from build123d import *

# Parameters (mm, degrees)
SKIZZE1_W                       = 50
SKIZZE1_H                       = 29
SKIZZE1_R                       = 3
AUFSATZ_LINEAR_AUSTRAGEN1_DEPTH = 2
SKIZZE2_W                       = 30
SKIZZE2_H                       = 2
AUFSATZ_LINEAR_AUSTRAGEN2_DEPTH = 49.5
SKIZZE3_R                       = 1.5
SKIZZE3_R_2                     = 1.822550398
SKIZZE3_W                       = 4
SKIZZE3_H                       = 11
SKIZZE3_W_2                     = 6.639290737
SKIZZE3_H_2                     = 4.5
SCHNITT_LINEAR_AUSTRAGEN1_DEPTH = 49.5
SKIZZE4_W                       = 20
SKIZZE4_H                       = 12.5
SCHNITT_LINEAR_AUSTRAGEN2_DEPTH = 49.5


with BuildPart() as part:
    # Skizze1 → Aufsatz-Linear austragen1 (new body)
    with BuildSketch(Plane(origin=(0, 0, 0), x_dir=(1, 0, 0), z_dir=(0, 1, 0))):
        Rectangle(SKIZZE1_W, SKIZZE1_H)
        with Locations(Location((14.802393345, -9.5, 0), (0, 0, 270))):
            Circle(SKIZZE1_R, mode=Mode.SUBTRACT)
        with Locations(Location((-17.197606655, -9.5, 0), (0, 0, 270))):
            Circle(SKIZZE1_R, mode=Mode.SUBTRACT)
    extrude(amount=AUFSATZ_LINEAR_AUSTRAGEN1_DEPTH)

    # Skizze2 → Aufsatz-Linear austragen2 (add)
    with BuildSketch(Plane(origin=(0, 2, 0), x_dir=(1, 0, 0), z_dir=(0, 1, 0))):
        with Locations((-10, 13.5)):
            Rectangle(SKIZZE2_W, SKIZZE2_H)
    extrude(amount=AUFSATZ_LINEAR_AUSTRAGEN2_DEPTH)

    # Skizze3 → Schnitt-Linear austragen1 (cut)
    with BuildSketch(Plane.XY.offset(-12.5)):
        with Locations((-22, 49)):
            Circle(SKIZZE3_R)
        with Locations((-22, 34)):
            Circle(SKIZZE3_R)
        with Locations((0, 41.5)):
            Circle(SKIZZE3_R_2)
        with Locations((-23, 41.5)):
            Rectangle(SKIZZE3_W, SKIZZE3_H)
        with Locations((-11.748940962, 49.25)):
            Rectangle(SKIZZE3_W_2, SKIZZE3_H_2)
    extrude(amount=-SCHNITT_LINEAR_AUSTRAGEN1_DEPTH, mode=Mode.SUBTRACT)

    # Skizze4 → Schnitt-Linear austragen2 (cut)
    with BuildSketch(Plane(origin=(0, 2, 0), x_dir=(1, 0, 0), z_dir=(0, 1, 0))):
        with Locations((15, 8.25)):
            Rectangle(SKIZZE4_W, SKIZZE4_H)
    extrude(amount=-SCHNITT_LINEAR_AUSTRAGEN2_DEPTH, mode=Mode.SUBTRACT)


solid = part.part
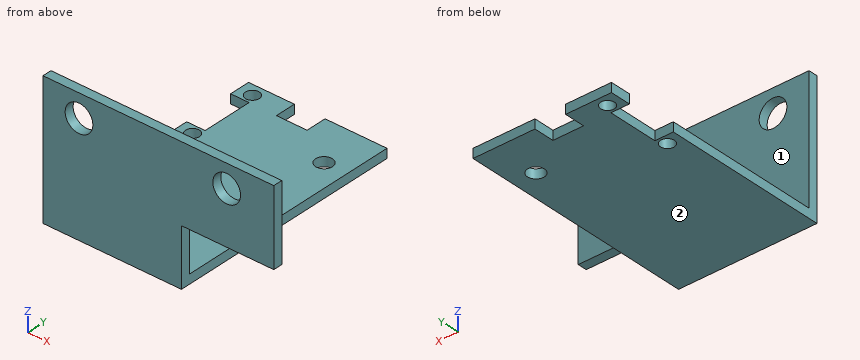
Design review of the part built by this model. Coordinates are the model's own, in mm. Face numbers are marked on the shaded views. A direction names the side the tool comes from. Coordinates: 2 decimals unless noted, no trailing zeros. Loops run counter-clockwise (first coordinate to the right, second up) from the corner with the lowest first, then second, coordinate; pieces in that order, holes last.
Item 1: Add section A-A (y = 41.5). Write out the cut boundary in (x, z), and give its area (3 significant figures).
Completed:
outline: (-21, -14.5) - (-1.82, -14.5) - (-1.82, -12.5) - (-21, -12.5) - close; (1.82, -14.5) - (5, -14.5) - (5, -12.5) - (1.82, -12.5) - close
area: 44.7 mm2
Item 2: Add section C-C (x = -22). Write out the cut boundary in (y, z), and give its area (3 significant figures).
Completed:
outline: (0, -14.5) - (32.5, -14.5) - (32.5, -12.5) - (2, -12.5) - (2, 14.5) - (0, 14.5) - close; (35.5, -14.5) - (36, -14.5) - (36, -12.5) - (35.5, -12.5) - close; (47, -14.5) - (47.5, -14.5) - (47.5, -12.5) - (47, -12.5) - close; (50.5, -14.5) - (51.5, -14.5) - (51.5, -12.5) - (50.5, -12.5) - close
area: 123 mm2
Item 3: For the marked faces 1 and 2, list the 3-axis set-ups (+Z, -Z, +X, -X, +Y, -Y) from which the entire face can be reached by the end or side of a thin tool; tool diameter is ignored.
Completed:
face 1: +Z, +X, -X, +Y
face 2: -Z, +X, -X, +Y, -Y
Item 4: Clearance check with flat-ended pins moving along their axes: pin 1 (8 mm diameter, centred on x = -5.5, y = 13, fed in from +Z); pin 2 (1 mm diameter, centred on x = 12.5, z = 10, fed in from -Y); pin 3 (9.5 mm diameter, centred on x = 14.8, z = 9.5, fed in from +Y); pin 4 (1 mm diameter, centred on x = 10, y = 1.5, fed in from -Z). State where each tip first meets the part, or that it passes through.
Completed:
pin 1: stops at z = -12.5
pin 2: passes through
pin 3: stops at y = 2
pin 4: stops at z = -2
Item 5: Add section B-B (z = 9.5). Write out the cut boundary in (x, y), and give its area (3 significant figures).
Completed:
outline: (-25, 0) - (-20.2, 0) - (-20.2, 2) - (-25, 2) - close; (-14.2, 0) - (11.8, 0) - (11.8, 2) - (-14.2, 2) - close; (17.8, 0) - (25, 0) - (25, 2) - (17.8, 2) - close
area: 76.0 mm2
Item 6: Add section D-D (y = 49). Write out the cut boundary in (x, z).
Completed:
outline: (-25, -14.5) - (-23.5, -14.5) - (-23.5, -12.5) - (-25, -12.5) - close; (-20.5, -14.5) - (-15.07, -14.5) - (-15.07, -12.5) - (-20.5, -12.5) - close; (-8.43, -14.5) - (5, -14.5) - (5, -12.5) - (-8.43, -12.5) - close
Item 7: Wall thickness on L1, parallel to Y at x = -22, z = -13.2; L2, parallel to Y at x = 9, z = 7; L3, parallel to Z at x = -8.5, y = 14: over which ranges is each line inside the solid? List them lowest first.
Completed:
L1: y = 0 to 32.5, 35.5 to 36, 47 to 47.5, 50.5 to 51.5
L2: y = 0 to 2
L3: z = -14.5 to -12.5
